For this review, use the dimensioned drawing (mm, ordinates from the lowest corner) and the shaded views. A direction names the side the tool comes from. Round coordinates to 2 decimals unless told otherwise and drop trailing zeros. Order: outer loops, then holes, each group sorted by start corner. A loop starts at its lowest first (then second) coordinate and runs counter-clockwise, first axis right, second up. Notation, with made-up numbers: M 46,32 L 63,32 A15 cw 63,46 Z; hole C 44.5,-29 d1. An arc over 180 degrees is marked long. Use a Markdown table: item, result. Add a question column.
1. For the marked faces 4, 5 and 6, list the 3-axis set-ups (+Z, -Z, +X, -X, +Y, -Y) from which the entire face can be reached by the end or side of a thin tool; tool diameter is ignored.
2. Consider section A-A on y = 31.77. State the section outline as (x, z) points (3 decimals), then the cut area to 3 significant figures.
3. To check wall thickness, follow probe 1 along Y at (x, z) = (27, 2.5); probe 2 along X at (y, z) = (11, 3); probe 3 along X at (y, z) = (4.5, 4.25). State the ranges of each line that lie inside material, in increasing order.
4. Insertion check: P1, Ø6, axis at x = 22, y = 17.5, coming from the -Z side; P2, Ø4, axis at x = 22, z = 4.5, coming from the +Y side; P3, Ø3.5, axis at x = 3.585, y = 3.83, coming from the -Z side. Each pin has a flat end and moves straight along its axis. Give the tip position at first contact, or say it passes through.
5. Consider section C-C on x = 29.5. State the section outline as (y, z) points.
6. Consider section D-D on y = 3.83. State the section outline as (x, z) points (3 decimals), then the cut area to 3 significant figures.
7. The part is to be moulded in two halves that separate along X. For the marked faces 1, 2 and 3, say which applies: +X half, -X half, draft (parallel to the pull), parting line (faces both ways), or undercut.
8. Consider section B-B on z = 5. State the section outline as (x, y) points (3 decimals), then the cut area to 3 significant figures.
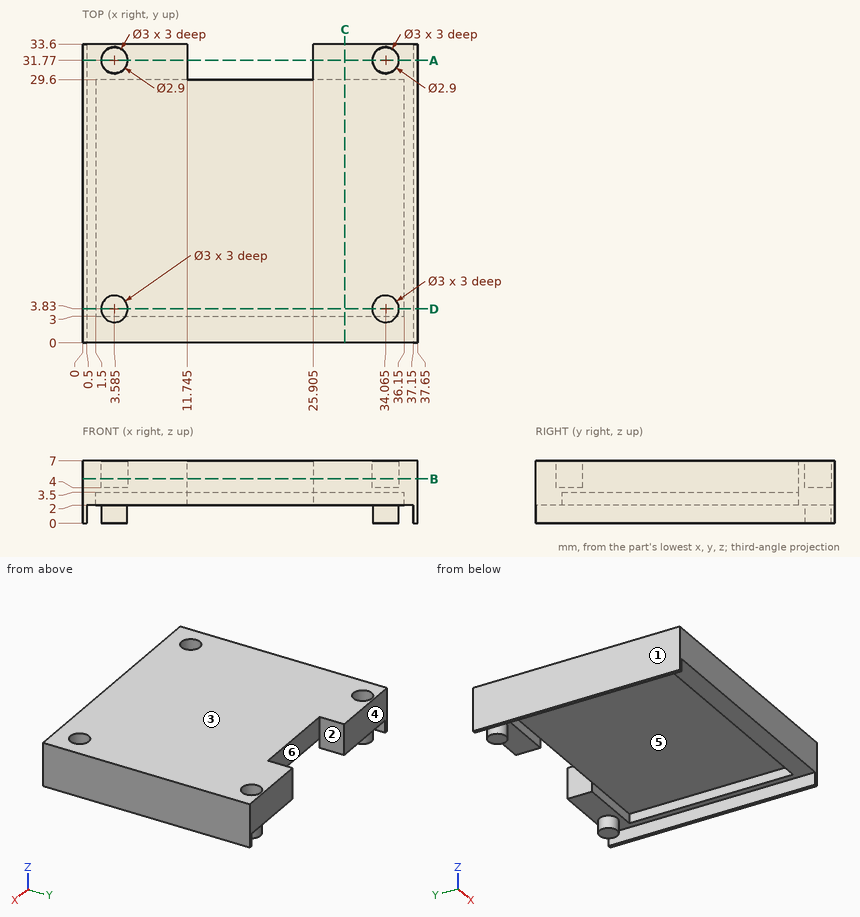
Answer block:
| question | item | result |
|---|---|---|
| 1 | face 4 | +Z, -Z, +X, -X, +Y |
| 1 | face 5 | -Z |
| 1 | face 6 | +Z, -Z, +Y |
| 2 | outline | M 0,0 L 0.5,0 L 0.5,2 L 2.135,2 L 2.135,0 L 5.035,0 L 5.035,2 L 11.745,2 L 11.745,7 L 5.085,7 L 5.085,4 L 2.085,4 L 2.085,7 L 0,7 Z; M 25.905,2 L 32.615,2 L 32.615,0 L 35.515,0 L 35.515,2 L 37.15,2 L 37.15,0 L 37.65,0 L 37.65,7 L 35.565,7 L 35.565,4 L 32.565,4 L 32.565,7 L 25.905,7 Z |
| 2 | area | 113 mm^2 |
| 3 | probe 1 | 0 to 3, 29.6 to 33.6 |
| 3 | probe 2 | 0 to 1.5, 36.15 to 37.65 |
| 3 | probe 3 | 0 to 2.24, 4.93 to 32.72, 35.41 to 37.65 |
| 4 | P1 | z = 3.5 |
| 4 | P2 | y = 29.6 |
| 4 | P3 | z = 2 |
| 5 | outline | M 0,2 L 3,2 L 3,3.5 L 29.6,3.5 L 29.6,2 L 33.6,2 L 33.6,7 L 0,7 Z |
| 6 | outline | M 0,0 L 0.5,0 L 0.5,2 L 1.5,2 L 1.5,3.5 L 36.15,3.5 L 36.15,2 L 37.15,2 L 37.15,0 L 37.65,0 L 37.65,7 L 35.565,7 L 35.565,4 L 32.565,4 L 32.565,7 L 5.085,7 L 5.085,4 L 2.085,4 L 2.085,7 L 0,7 Z |
| 6 | area | 120 mm^2 |
| 7 | face 1 | -X half |
| 7 | face 2 | undercut |
| 7 | face 3 | draft |
| 8 | outline | M 0,0 L 37.65,0 L 37.65,33.6 L 25.905,33.6 L 25.905,29.6 L 11.745,29.6 L 11.745,33.6 L 0,33.6 Z; hole C 3.585,3.83 d3; hole C 3.585,31.77 d3; hole C 34.065,3.83 d3; hole C 34.065,31.77 d3 |
| 8 | area | 1,180 mm^2 |
